```python
from build123d import *

# Parameters (mm, degrees)
F1_DEPTH = 25.4
F2_DEPTH = 12.7
F4_DEPTH = 25.4


# Not quite as in the source:
# - the program builds the solid bodies; features that only make, move or delete a surface that nothing else refers to are left out


with BuildPart() as f1:
    # F0 (on Front) → F1 (new body)
    with BuildSketch(Plane.XZ):
        Polygon((-22.1610441804, -43.1708656251), (0, -43.1708656251), (22.1610441804, -43.1708656251), (35.4001075029, -30.2196051925), (35.4001075029, 31.3708260655), (26.4781303704, 44.897697866), (0, 44.897697866), (-26.4781303704, 44.897697866), (-35.4001075029, 31.3708260655), (-35.4001075029, -30.2196051925), align=None)
    extrude(amount=F1_DEPTH)

    # F2 (cut): a face of the model
    f2_faces = [f1.faces().sort_by_distance(p)[0] for p in [
        (0, -25.4, 1.2066431814),
    ]]
    extrude(f2_faces, amount=-F2_DEPTH, mode=Mode.SUBTRACT)

    # F3 (on Front) → F4 (join)
    with BuildSketch(Plane.XZ):
        Polygon((34.8244979978, 49.5025888085), (0, 49.5025888085), (-34.8244979978, 49.5025888085), (-43.1708618999, 0), (-35.4001075029, -50.3660067916), (0, -50.3660067916), (35.4001075029, -50.3660067916), (43.1708618999, 0), align=None)
    extrude(amount=-F4_DEPTH)


solid = f1.part
```
The listing builds one solid part. Answer for the finished solid, in the listing's coordinates (mm). A direction names the side the tool comes from. Coordinates: 2 decimals unless noted, no trailing zeros. Write each loop counter-clockwise with the first axis right and the second up, starting at its lowest first coordinate (ties: lowest second). Pieces come first, ordered by that corner, then holes.
Q1. Section B-B, the plane x = 7.5 is taken. Write down the section's boundary in (y, z), then the cut area to 3 significant figures.
Returned:
outline: (-12.7, -43.17) - (0, -43.17) - (0, -50.37) - (25.4, -50.37) - (25.4, 49.5) - (0, 49.5) - (0, 44.9) - (-12.7, 44.9) - close
area: 3,660 mm2
Q2. Given P1, Ø4, axis at y = 11.5, z = -12.5, coming from the -X side; P2, Ø14, axis at y = -6.5, z = 11, coming from the -X side; P3, Ø8, axis at y = 2.5, z = 7, coming from the -X side, each flat-ended and moving along its own axis, determine where each tip first touches the part or whether it passes through.
Returned:
P1: stops at x = -41.55
P2: stops at x = -41.75
P3: stops at x = -42.67
Q3. Section A-A, the plane y = -10 is taken. Write down the section's boundary in (x, z), then the cut area to 3 significant figures.
Returned:
outline: (-35.4, -30.22) - (-22.16, -43.17) - (22.16, -43.17) - (35.4, -30.22) - (35.4, 31.37) - (26.48, 44.9) - (-26.48, 44.9) - (-35.4, 31.37) - close
area: 5,940 mm2
Q4. Section C-C, the plane y = 8 is taken. Write down the section's boundary in (x, z).
Returned:
outline: (-43.17, 0) - (-35.4, -50.37) - (35.4, -50.37) - (43.17, 0) - (34.82, 49.5) - (-34.82, 49.5) - close
Q5. Find the intervals of material crossed by line 1 along X through (y, z) = (-2.5, -3.5); line 2 along Y through (x, z) = (37.5, -30); line 3 along Z through (x, y) = (-11.5, -4), in increasing order.
Returned:
line 1: x = -35.4 to 35.4
line 2: y = 0 to 25.4
line 3: z = -43.17 to 44.9
Q6. Which of the six approach directions +Z, -Z, +X, -X, +Y, -Y give full straight-line access (tool end or side, diameter ignored) to faces 1 (the flat face through (35.4, -6, 0)), 2 (the flat face through (0, -6, 44.898)), 3 (the flat face through (31, -6.26, 38.04)), 4 (the flat face through (0, 0, -45)), 5 (the flat face through (-30.877, -6.261, 38.229))?
Returned:
face 1: +Z, -Z, +X, -Y
face 2: +Z, +X, -X, -Y
face 3: +Z, +X, -Y
face 4: -Y
face 5: +Z, -X, -Y
